Could you check a few things on this model? Use its own coordinates, in mm. A direction names the side the tool comes from. Coordinates: 2 decimals unless noted, no trailing zeros. Write each loop counter-clockwise with the first axis right and the second up, starting at its lowest first coordinate (ties: lowest second). Pieces come first, ordered by that corner, then holes.
Item 1: Thinking about a two-plate mould opening in Z: for faces 3 (the cylindrical face through (30, 2, 10.4)), 4 (the cylindrical face through (41, 2.03, -16.07)), 5 (the cylindrical face through (-31.781, 2.028, 17.127)), which applies, +Z half, -Z half, draft (parallel to the pull), parting line (faces both ways), or undercut?
Item 2: If I drill on probe 1 along X at (y, z) = (2.6, -9.5); probe 2 along Z at (x, y) = (0, 2.2); probe 3 along X at (y, z) = (2.25, 10.5), over which ranges is the centre line in solid material (lowest first)?
Item 3: I want a section at C-C on z = -9.5. Please give me the cut outline in (x, y), then the cut area to 3 significant figures.
Item 4: I want a section at B-B on y = 1.1. Please give me the cut outline in (x, z), then the cut area to 3 significant figures.
Item 5: I want a section at D-D on z = 5.5. Please give me the cut outline in (x, y), then the cut area to 3 significant figures.
Item 6: I want a section at A-A on x = 0. Please give me the cut outline in (y, z).
Item 7: Which directions (+Z, -Z, +X, -X, +Y, -Y) give clear straight access to the entire face, cutting with the end or side of a thin tool? Please do faces 1 (the cylindrical face through (31.73, 2.028, 17.106)), 2 (the flat face through (-36, 2, 17.5)).
from build123d import *

# Parameters (mm, degrees)
SKETCH1_R           = 3
SKETCH1_R_2         = 4.05
BOSS_EXTRUDE1_DEPTH = 4
FILLET1_R           = 5


with BuildPart() as part:
    # Sketch1 → Boss-Extrude1 (new body)
    with BuildSketch(Plane(origin=(0, 0, 0), x_dir=(1, 0, 0), z_dir=(0, 1, 0))):
        with BuildLine():
            Line((-42.5, 17.5), (-42.5, -17.5))
            Line((-42.5, -17.5), (-31.527765541, -17.5))
            ThreePointArc((-31.527765541, -17.5), (0, -3.5), (31.527765541, -17.5))
            Line((31.527765541, -17.5), (42.5, -17.5))
            Line((42.5, -17.5), (42.5, 17.5))
            Line((42.5, 17.5), (-42.5, 17.5))
        make_face()
        with Locations((-33, -10.5)):
            Circle(SKETCH1_R, mode=Mode.SUBTRACT)
        with Locations((-33, 9.5)):
            Circle(SKETCH1_R_2, mode=Mode.SUBTRACT)
        with Locations((33, -10.5)):
            Circle(SKETCH1_R, mode=Mode.SUBTRACT)
        with Locations((0, 9.5)):
            Circle(SKETCH1_R_2, mode=Mode.SUBTRACT)
        with Locations((33, 9.5)):
            Circle(SKETCH1_R_2, mode=Mode.SUBTRACT)
    extrude(amount=BOSS_EXTRUDE1_DEPTH)

    # Fillet1
    fillet1_edges = [part.edges().sort_by_distance(p)[0] for p in [
        (-31.527765541, 2, 17.5),
        (-42.5, 2, 17.5),
        (-42.5, 2, -17.5),
        (42.5, 2, -17.5),
        (42.5, 2, 17.5),
        (31.527765541, 2, 17.5),
    ]]
    fillet(fillet1_edges, radius=FILLET1_R)


solid = part.part
Response values:
1. face 3: undercut
1. face 4: -Z half
1. face 5: +Z half
2. probe 1: x = -42.5 to -37.05, -28.95 to -4.05, 4.05 to 28.95, 37.05 to 42.5
2. probe 2: z = -17.5 to -13.55, -5.45 to 3.5
2. probe 3: x = -42.5 to -36, -30 to -23.37, 23.37 to 30, 36 to 42.5
3. outline: (-42.5, 0) - (-37.05, 0) - (-37.05, 4) - (-42.5, 4) - close; (-28.95, 0) - (-4.05, 0) - (-4.05, 4) - (-28.95, 4) - close; (4.05, 0) - (28.95, 0) - (28.95, 4) - (4.05, 4) - close; (37.05, 0) - (42.5, 0) - (42.5, 4) - (37.05, 4) - close
3. area: 243 mm2
4. outline: (-42.5, -12.5) arc R5 ccw to (-37.5, -17.5) - (37.5, -17.5) arc R5 ccw to (42.5, -12.5) - (42.5, 12.5) arc R5 ccw to (37.5, 17.5) - (33.67, 17.5) arc R5 ccw to (30.13, 16.03) arc R42.5 cw to (-30.13, 16.03) arc R5 ccw to (-33.67, 17.5) - (-37.5, 17.5) arc R5 ccw to (-42.5, 12.5) - close; hole circle Ø8.1 at (-33, -9.5); hole circle Ø6 at (-33, 10.5); hole circle Ø8.1 at (0, -9.5); hole circle Ø8.1 at (33, -9.5); hole circle Ø6 at (33, 10.5)
4. area: 2,130 mm2
5. outline: (-42.5, 0) - (-12.88, 0) - (-12.88, 4) - (-42.5, 4) - close; (12.88, 0) - (42.5, 0) - (42.5, 4) - (12.88, 4) - close
5. area: 237 mm2
6. outline: (0, -17.5) - (4, -17.5) - (4, -13.55) - (0, -13.55) - close; (0, -5.45) - (4, -5.45) - (4, 3.5) - (0, 3.5) - close
7. face 1: +Z, +Y, -Y
7. face 2: +Z, +X, -X, +Y, -Y
